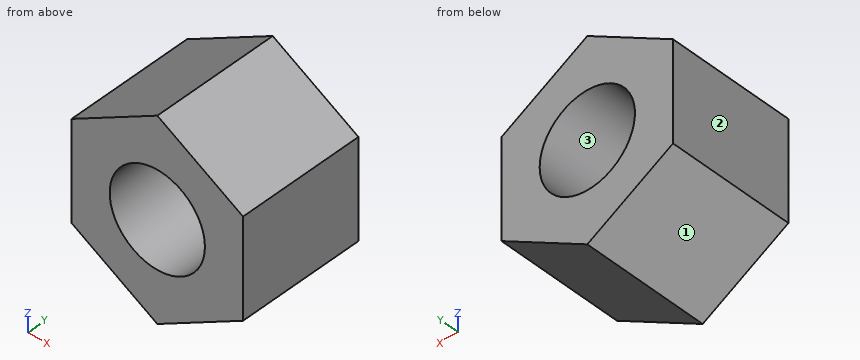
Autodesk Inventor part; units mm, degrees
ref_plane "YZ Plane" through (0, 0, 0) normal (1, 0, 0) x (0, 1, 0)
ref_plane "XZ Plane" through (0, 0, 0) normal (0, 1, 0) x (-1, 0, 0)
ref_plane "XY Plane" through (0, 0, 0) normal (0, 0, 1) x (1, 0, 0)
sketch "Sketch1" plane through (0, 0, 0) normal (0, 1, 0) x (-1, 0, 0)
  line L0 (0, -3.1177) -> (-2.7, -1.5588)
  line L1 (-2.7, -1.5588) -> (-2.7, 1.5588)
  line L2 (-2.7, 1.5588) -> (0, 3.1177)
  line L3 (0, 3.1177) -> (2.7, 1.5588)
  line L4 (2.7, 1.5588) -> (2.7, -1.5588)
  line L5 (2.7, -1.5588) -> (0, -3.1177)
  point P0 (0, 0)
  point P1 (0, 0)
  dimension "d0" = 5.4
extrude "Extrusion1" add sketch "Sketch1" along normal blind 4
sketch "Sketch2" plane through (0, 4, 0) normal (0, 1, 0) x (1, 0, 0)
  circle A0 centre (0, 0) radius 1.5
  dimension "d3" = 3
extrude "Extrusion2" cut sketch "Sketch2" against normal blind 4
properties part number "M3_lock_nut"
Could you check a few things on this model? Use its own coordinates, in mm. Face numbers are marked on the shaded views. Give positions to 0.01 mm unless a question says otherwise; leave off trailing zeros. Order: outer loops, then holes, each group sorted by start corner. A loop starts at its lowest first (then second) coordinate and runs counter-clockwise, first axis right, second up. Notation, with made-up numbers: (-17, 30.25) -> (34, 30.25) arc R10 cw to (34, 44.25) -> close; hole circle Ø6 at (-4.75, 76). An arc over 180 degrees is marked (long way). Answer in a Markdown table with one row per item. Add a question column.
Item 1: Imagine slicing it at A-A (z = 0). List the corners of the cut face in (x, y) for me, and give its area (3 significant figures).
Item 2: Imagine slicing it at D-D (x = 1.6). List the corners of the cut face in (y, z) for me, and give its area (3 significant figures).
Item 3: Imagine slicing it at C-C (x = -0.5). List the corners of the cut face in (y, z) for me, and give its area (3 significant figures).
Item 4: Please list where these lines run through material, in increasing order: probe 1 along X at (y, z) = (1.2, 0); probe 2 along Z at (x, y) = (-0.15, 2.55); probe 3 along Z at (x, y) = (1.3, 2.3).
Item 5: We'd pull the mould along Z, two halves only. Please class the marked faces 1, 2 and 3: pulls with the +Z half, pulls with the -Z half, needs draft (parallel to the pull), parting line crosses it, or undercut.
Item 6: Imagine slicing it at B-B (y = 2.6). List the corners of the cut face in (x, z) for me.
Item 7: I'm going to push flat-ended pins straight in: P1, Ø2, axis at x = -1.5, y = 3.5, coming from the -Z side; P2, Ø1, axis at y = 3.5, z = 2.5, coming from the +X side; P3, Ø2.5, axis at x = 0, z = 0, coming from the +Y side; P4, Ø1, axis at y = 3, z = 2.5, coming from the -X side. Where does each tip first touch, or does it pass through?
Result:
| question | item | result |
|---|---|---|
| 1 | outline | (-2.7, 0) -> (-1.5, 0) -> (-1.5, 4) -> (-2.7, 4) -> close; (1.5, 0) -> (2.7, 0) -> (2.7, 4) -> (1.5, 4) -> close |
| 1 | area | 9.60 mm2 |
| 2 | outline | (0, -2.19) -> (4, -2.19) -> (4, 2.19) -> (0, 2.19) -> close |
| 2 | area | 17.6 mm2 |
| 3 | outline | (0, -2.83) -> (4, -2.83) -> (4, -1.41) -> (0, -1.41) -> close; (0, 1.41) -> (4, 1.41) -> (4, 2.83) -> (0, 2.83) -> close |
| 3 | area | 11.3 mm2 |
| 4 | probe 1 | -2.7 to -1.5, 1.5 to 2.7 |
| 4 | probe 2 | -3.03 to -1.49, 1.49 to 3.03 |
| 4 | probe 3 | -2.37 to -0.75, 0.75 to 2.37 |
| 5 | face 1 | pulls with the -Z half |
| 5 | face 2 | needs draft |
| 5 | face 3 | undercut |
| 6 | outline | (-2.7, -1.56) -> (0, -3.12) -> (2.7, -1.56) -> (2.7, 1.56) -> (0, 3.12) -> (-2.7, 1.56) -> close; hole circle Ø3 at (0, 0) |
| 7 | P1 | z = -2.83 |
| 7 | P2 | x = 1.94 |
| 7 | P3 | through |
| 7 | P4 | x = -1.94 |
